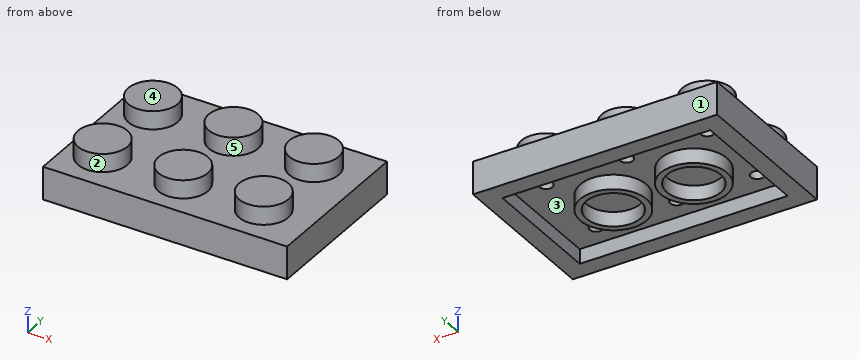
from build123d import *

# Parameters (mm, degrees)
F0_W      = 23.876
F0_H      = 15.748
F1_DEPTH  = 3.20802
F2_R      = 2.413
F3_DEPTH  = 1.778
F2_R_2    = 2.4164208991
F4_DEPTH  = 1.778
F2_R_3    = 2.4201182345
F5_DEPTH  = 1.778
F6_DEPTH  = 1.778
F7_DEPTH  = 1.778
F8_DEPTH  = 1.778
F9_T      = -1.778
F10_R     = 3.2385
F10_R_2   = 2.6416
F11_DEPTH = 3.06898


# Not quite as in the source:
# - a feature names something its author has since deleted; it is built from what else it names


with BuildPart() as f1:
    # F0 (on Top) → F1 (new body)
    with BuildSketch(Plane.XY):
        with Locations((11.938, 7.874)):
            Rectangle(F0_W, F0_H)
    extrude(amount=F1_DEPTH)

    # F2 (on face) → F3 (join)
    with BuildSketch(Plane.XY.offset(3.20802)):
        with Locations((3.3980837251, 11.858843371)):
            Circle(F2_R)
    extrude(amount=F3_DEPTH)

    # F2 (on face) → F4 (join)
    with BuildSketch(Plane.XY.offset(3.20802)):
        with Locations((11.2720837251, 11.858843371)):
            Circle(F2_R_2)
    extrude(amount=F4_DEPTH)

    # F2 (on face) → F5 (join)
    with BuildSketch(Plane.XY.offset(3.20802)):
        with Locations((19.1460837251, 11.858843371)):
            Circle(F2_R_3)
    extrude(amount=F5_DEPTH)

    # F2 (on face) → F6 (join)
    with BuildSketch(Plane.XY.offset(3.20802)):
        with Locations((3.3980837251, 3.9364123053)):
            Circle(F2_R)
    extrude(amount=F6_DEPTH)

    # F2 (on face) → F7 (join)
    with BuildSketch(Plane.XY.offset(3.20802)):
        with Locations((11.2720837251, 3.9364123053)):
            Circle(F2_R)
    extrude(amount=F7_DEPTH)

    # F2 (on face) → F8 (join)
    with BuildSketch(Plane.XY.offset(3.20802)):
        with Locations((19.1460837251, 3.9364123053)):
            Circle(F2_R)
    extrude(amount=F8_DEPTH)

    # F9
    f9_openings = [f1.faces().sort_by_distance(p)[0] for p in [
        (11.938, 7.874, 0),
    ]]
    offset(amount=F9_T, openings=f9_openings, kind=Kind.INTERSECTION)

    # F10 (on face) → F11 (join)
    with BuildSketch(Plane.XY):
        with BuildLine():
            ThreePointArc((4.1275, 7.5388690457), (7.366, 4.3003690457), (10.6045, 7.5388690457))
            ThreePointArc((10.6045, 7.5388690457), (7.366, 10.7773690457), (4.1275, 7.5388690457))
        make_face()
        with BuildLine():
            ThreePointArc((10.0076, 7.5388690457), (7.366, 4.8972690457), (4.7244, 7.5388690457))
            ThreePointArc((4.7244, 7.5388690457), (7.366, 10.1804690457), (10.0076, 7.5388690457))
        make_face(mode=Mode.SUBTRACT)
        with Locations((15.24, 7.5388690457)):
            Circle(F10_R)
        with Locations((15.24, 7.5388690457)):
            Circle(F10_R_2, mode=Mode.SUBTRACT)
    extrude(amount=F11_DEPTH)


solid = f1.part
Geometry check sheet. Reference: the model listing, model coordinates, mm. Face numbers are marked on the shaded views. A direction names the side the tool comes from. Coordinates: 2 decimals unless noted, no trailing zeros. Order: outer loops, then holes, each group sorted by start corner. A loop starts at its lowest first (then second) coordinate and runs counter-clockwise, first axis right, second up. Notation, with made-up numbers: (-33.5, 47.25) -> (21.5, 47.25) arc R21 ccw to (21.5, 70.25) -> close; hole circle Ø7 at (22, 87). An arc over 180 degrees is marked (long way). Use a Markdown table: item, result. Add a question column.
1. Go/stop test with flat-tipped pins: pin 1 Ø1.4 at (x, y) = (19, 12) entering from -Z; pin 2 Ø0.6 at (x, y) = (3.5, 12) entering from -Z. Record where each tip stops, or that it passes through.
2. Material ranges on L1, parallel to Y at x = 15.24, z = 0.45; L2, parallel to X at y = 4, z = 0.35; L3, parallel to X at y = 7, z = 0.55, recorded low to high.
3. Set-up check for the marked faces 1, 2 and 3: record each of +Z, -Z, +X, -X, +Y, -Y from which the full face is reachable in a straight line by a thin tool's end or side.
4. Cross-section at A-A (z = 1.05). Enter the section's corners in (x, y), and give its area (3 significant figures).
5. Mould release check, pull along X, two halves, no side actions. Record for the marked faces 4 and 5: pulls with the +X half, pulls with the -X half, needs draft (parallel to the pull), parting line crosses it, or undercut.
6. Cross-section at B-B (x = 15.24). Enter the section's corners in (y, z).
7. Cross-section at D-D (x = 19.5). Enter the section's corners in (y, z), and give its area (3 significant figures).
8. Cross-section at C-C (z = 3.55). Enter the section's corners in (x, y).
Filled sheet:
| question | item | result |
|---|---|---|
| 1 | pin 1 | z = 1.43 |
| 1 | pin 2 | z = 3.21 |
| 2 | L1 | 0 to 1.78, 4.3 to 4.9, 10.18 to 10.78, 13.97 to 15.75 |
| 2 | L2 | 0 to 1.78, 22.1 to 23.88 |
| 2 | L3 | 0 to 1.78, 4.17 to 4.78, 9.95 to 10.56, 12.05 to 12.65, 17.83 to 18.43, 22.1 to 23.88 |
| 3 | face 1 | +Z, -Z, +X, -X, +Y |
| 3 | face 2 | +Z |
| 3 | face 3 | -Z |
| 4 | outline | (0, 0) -> (23.88, 0) -> (23.88, 15.75) -> (0, 15.75) -> close; circle Ø6.48 at (7.37, 7.54); circle Ø6.48 at (15.24, 7.54); hole (1.78, 1.78) -> (22.1, 1.78) -> (22.1, 13.97) -> (1.78, 13.97) -> close; hole circle Ø5.28 at (7.37, 7.54); hole circle Ø5.28 at (15.24, 7.54) |
| 4 | area | 150 mm2 |
| 5 | face 4 | needs draft |
| 5 | face 5 | undercut |
| 6 | outline | (0, 0) -> (1.78, 0) -> (1.78, 1.43) -> (4.3, 1.43) -> (4.3, 0) -> (4.9, 0) -> (4.9, 1.43) -> (10.18, 1.43) -> (10.18, 0) -> (10.78, 0) -> (10.78, 1.43) -> (13.97, 1.43) -> (13.97, 0) -> (15.75, 0) -> (15.75, 3.21) -> (0, 3.21) -> close |
| 7 | outline | (0, 0) -> (1.78, 0) -> (1.78, 1.43) -> (3.41, 1.43) -> (3.41, 3.21) -> (4.46, 3.21) -> (4.46, 1.43) -> (11.32, 1.43) -> (11.32, 3.21) -> (12.39, 3.21) -> (12.39, 1.43) -> (13.97, 1.43) -> (13.97, 0) -> (15.75, 0) -> (15.75, 3.21) -> (14.25, 3.21) -> (14.25, 4.99) -> (9.46, 4.99) -> (9.46, 3.21) -> (6.32, 3.21) -> (6.32, 4.99) -> (1.55, 4.99) -> (1.55, 3.21) -> (0, 3.21) -> close |
| 7 | area | 46.3 mm2 |
| 8 | outline | circle Ø4.83 at (3.4, 3.94); circle Ø4.83 at (3.4, 11.86); circle Ø4.83 at (11.27, 3.94); circle Ø4.83 at (11.27, 11.86); circle Ø4.83 at (19.15, 3.94); circle Ø4.84 at (19.15, 11.86) |
